```python
from build123d import *

# Parameters (mm, degrees)
SKETCH_1_W          = 160
SKETCH_1_H          = 30
EXTRUDE_1_DEPTH     = 5
SKETCH_2_R          = 15
EXTRUDE_2_DEPTH     = 5
SKETCH_3_R          = 5
SKETCH_3_R_2        = 4
CUT_EXTRUDE_1_DEPTH = 6
SKETCH_4_W          = 15
SKETCH_4_H          = 5
EXTRUDE_3_DEPTH     = 3


with BuildPart() as part:
    # 草图1 → 凸台-拉伸1 (new body)
    with BuildSketch(Plane.XY):
        Rectangle(SKETCH_1_W, SKETCH_1_H)
    extrude(amount=EXTRUDE_1_DEPTH)

    # 草图2 → 凸台-拉伸2 (add)
    with BuildSketch(Plane.XY.offset(5)):
        with Locations((-60, -15)):
            Circle(SKETCH_2_R)
        with Locations((77, -15)):
            Circle(SKETCH_2_R)
    extrude(amount=-EXTRUDE_2_DEPTH)

    # 草图3 → 切除-拉伸1 (cut, through all)
    with BuildSketch(Plane.XY.offset(5)):
        with Locations((-60, -15)):
            Circle(SKETCH_3_R)
        with Locations((77, -15)):
            Circle(SKETCH_3_R_2)
    extrude(amount=-CUT_EXTRUDE_1_DEPTH, mode=Mode.SUBTRACT)

    # 草图4 → 凸台-拉伸3 (add)
    with BuildSketch(Plane(origin=(0, 15, 0), x_dir=(1, 0, 0), z_dir=(0, 1, 0))):
        with Locations((35.5, -2.5)):
            Rectangle(SKETCH_4_W, SKETCH_4_H)
    extrude(amount=EXTRUDE_3_DEPTH)


solid = part.part
```
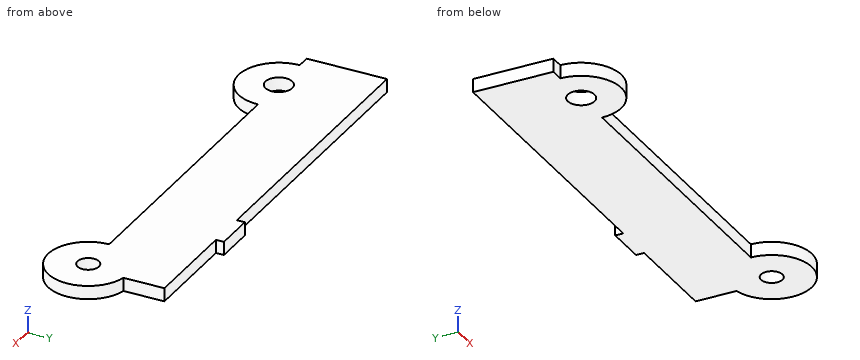
Read the model definition and answer for the solid it produces. Units are mm, in the model's axes. Give positions to 0.01 mm unless a question says otherwise; leave off trailing zeros. Write each loop counter-clockwise with the first axis right and the second up, starting at its lowest first coordinate (ties: lowest second). Pieces come first, ordered by that corner, then holes. Notation, with made-up numbers: (-35.75, 76.25) - (-21.75, 76.25) arc R28 cw to (-21.75, 114.25) - close; hole circle Ø10 at (24, 22). An arc over 180 degrees is marked (long way). Write item = value, one per line. Start each with the question number.
Item 1: Find section A-A (x = -60). Give the vertices of the cut face in (y, z), then the cut area to 3 significant figures.
Item 2: Find section D-D (y = -17). Give the vertices of the cut face in (x, z), then the cut area to 3 significant figures.
Item 3: Each of these flat-tipped pins is pushed along its axis until it touches: P1, Ø1.5, axis at x = 67, z = 2, coming from the +Y side; P2, Ø1, axis at x = -49.5, z = 3, coming from the -Y side; P3, Ø0.9, axis at y = 16.5, z = 3, coming from the +X side. Where does it stop, or does it pass through?
Item 4: Find section B-B (y = -25.5). Give the vertices of the cut face in (x, z), then the cut area to 3 significant figures.
Item 5: Find section C-C (z = 3). Give the vertices of the cut face in (x, y), then the cut area to 3 significant figures.
Item 6: Find the intervals of material crossed by probe 1 along X at (y, z) = (-19.5, 2.9); probe 2 along Y at (x, z) = (-60, 1.45); probe 3 along Y at (x, z) = (77, 1.85), in increasing order. Write a range as [from, to].
Response:
q1.outline = (-30, 0) - (-20, 0) - (-20, 5) - (-30, 5) - close; (-10, 0) - (15, 0) - (15, 5) - (-10, 5) - close
q1.area = 175 mm²
q2.outline = (-74.87, 0) - (-64.58, 0) - (-64.58, 5) - (-74.87, 5) - close; (-55.42, 0) - (-45.13, 0) - (-45.13, 5) - (-55.42, 5) - close; (62.13, 0) - (73.54, 0) - (73.54, 5) - (62.13, 5) - close; (80.46, 0) - (91.87, 0) - (91.87, 5) - (80.46, 5) - close
q2.area = 217 mm²
q3.P1 = 15
q3.P2 = -26.18
q3.P3 = 43
q4.outline = (-70.71, 0) - (-49.29, 0) - (-49.29, 5) - (-70.71, 5) - close; (66.29, 0) - (87.71, 0) - (87.71, 5) - (66.29, 5) - close
q4.area = 214 mm²
q5.outline = (-80, -15) - (-75, -15) arc R15 ccw to (-45, -15) - (62, -15) arc R15 ccw (long way) to (80, -0.3) - (80, 15) - (43, 15) - (43, 18) - (28, 18) - (28, 15) - (-80, 15) - close; hole circle Ø10 at (-60, -15); hole circle Ø8 at (77, -15)
q5.area = 5,560 mm²
q6.probe_1 = [-74.31, -62.18], [-57.82, -45.69], [62.69, 91.31]
q6.probe_2 = [-30, -20], [-10, 15]
q6.probe_3 = [-30, -19], [-11, 15]
